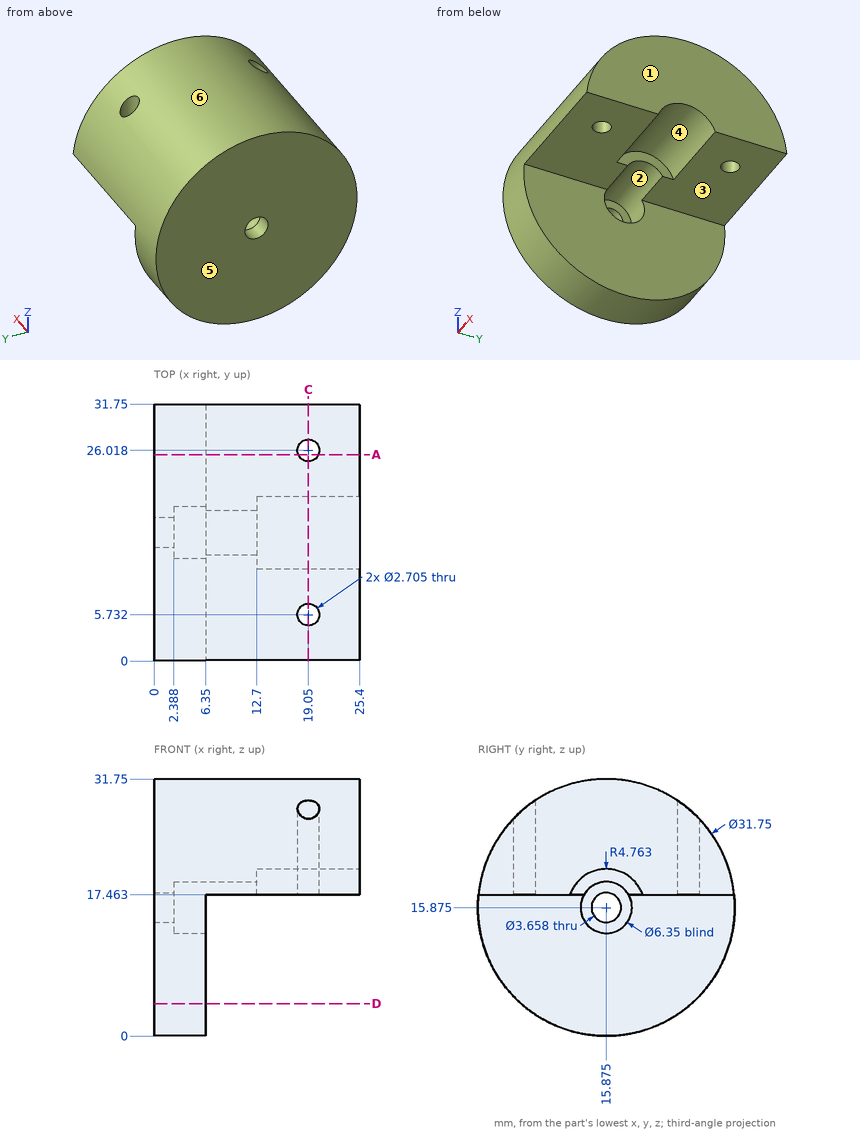
The figure shows three views and two pictorial views of one solid part (mm, origin at its lowest corner). Answer the questions. A direction names the side the tool comes from. Round coordinates to 2 decimals unless told otherwise and drop trailing zeros. Loops run counter-clockwise (first coordinate to the right, second up) from the corner with the lowest first, then second, coordinate; pieces in that order, holes last. Notation, with made-up numbers: M -9,-25 L 18,-25 A30 cw 18,10 Z; hole C 9,-8.75 d7. An arc over 180 degrees is marked long. Return JSON: item names as keys, results as strings.
Q1. The mould has two halves that part along Y. Classify the marked faces 4, 5 and 6: released by +Y, released by -Y, zero draft, split by the parting line, or undercut.
Results list:
{"face 4": "undercut", "face 5": "zero draft", "face 6": "split by the parting line"}
Q2. Find section D-D, the plane z = 4. Determine the outline of the cut face in (x, y), plus the area to 3 significant figures.
Results list:
{"outline": "M 0,5.34 L 6.35,5.34 L 6.35,26.41 L 0,26.41 Z", "area": "134 mm2"}
Q3. Find the intervals of material crossed by line 1 along Y through (x, z) = (19.05, 26.25) (1 decimal); line 2 along Z through (x, y) = (6, 17) (1 decimal); line 3 along Y through (x, z) = (19.75, 24) (1 decimal), in increasing order. Write a range as from..to.
Results list:
{"line 1": "y = 3.9..4.4, 7.1..24.7, 27.4..27.9", "line 2": "z = 0..12.9, 18.8..31.7", "line 3": "y = 2.2..4.6, 6.9..24.9, 27.2..29.5"}
Q4. Each of these flat-tipped pins is pushed along its axis until it touches: pin 1 Ø14 at (y, z) = (18, 11) entering from +X; pin 2 Ø4.5 at (x, y) = (19.05, 5.73) entering from +Z; pin 3 Ø5 at (x, z) = (6.5, 21.5) entering from +Y; pin 4 Ø4 at (x, y) = (10.5, 23) entering from +Z. Where does it stop, or does it pass through?
Results list:
{"pin 1": "stops at x = 25.4", "pin 2": "stops at z = 29.65", "pin 3": "stops at y = 31.44", "pin 4": "stops at z = 30.9"}
Q5. Find section A-A, the plane y = 25.5. Determine the outline of the cut face in (x, z).
Results list:
{"outline": "M 0,3.25 L 6.35,3.25 L 6.35,17.46 L 17.8,17.46 L 17.8,28.5 L 0,28.5 Z; M 20.3,17.46 L 25.4,17.46 L 25.4,28.5 L 20.3,28.5 Z"}
Q6. Which of the six approach directions +Z, -Z, +X, -X, +Y, -Y give full straight-line access (tool end or side, diameter ignored) to the marked faces 1, 2 and 3?
Results list:
{"face 1": "+Z, -Z, +X, +Y, -Y", "face 2": "+X", "face 3": "-Z, +X, +Y, -Y"}
Q7. Find section C-C, the plane x = 19.05. State how many separate pieces and enclosed holes the cut face has.
Results list:
{"separate pieces": "3", "enclosed holes": "0"}
